Part model, mm, in its own coordinate system. A direction names the side the tool comes from. Coordinates: 2 decimals unless noted, no trailing zeros. Loops run counter-clockwise (first coordinate to the right, second up) from the corner with the lowest first, then second, coordinate; pieces in that order, holes last. Notation, with made-up numbers: (6.5, -14.75) -> (31.5, -14.75) arc R26 cw to (31.5, -0.75) -> close; hole circle Ø7 at (-19, 72). An arc over 180 degrees is marked (long way). One line per question, with ' | ' between items. Start each with the question number.
1) Drop flat-ended pins along their axis: pin 1 (7.5 mm diameter, centred on y = 3, z = -0.5, fed in from -X); pin 2 (5 mm diameter, centred on x = 31, z = 0, fed in from +Y); pin 3 (4 mm diameter, centred on x = 14, z = -33, fed in from -Y); pin 4 (3.5 mm diameter, centred on x = 13.5, y = -12, fed in from -Z). Give the stop position or say it passes through.
2) Cut at C-C (x = -17.5). List the corners of the cut face in (y, z).
3) Cut at A-A (x = 0). List the corners of the cut face in (y, z), plus the area to 3 significant figures.
4) Cut at D-D (y = -1). List the corners of the cut face in (x, z), plus the area to 3 significant figures.
5) 3-axis set-ups, long thin cutter, end or side, ignore diameter. For faces 1 (the face through (23.5, 3, -42)), 2 (the face through (-32, 10, 5)), 3 (the face through (19.8, 11.51, 9.66)), 4 (the face through (-6, 2, -8)): which of +Z, -Z, +X, -X, +Y, -Y reach the whole face in a straight line?
6) Probe L1, parallel to Y at x = 0, z = -56.35; L2, parallel to X at y = 10, z = -55; L3, parallel to Y at x = 0, z = -39. List the from-to ranges inside material, lowest first. Write a range as from..to.
7) Cut at B-B (z = 6). List the corners of the cut face in (x, y).
8) Two-plate mould, pull along Y, no slides. Class faces 5 (the face through (6, 2, -9)), 6 (the face through (20, 11, -9)), 7 (the face through (0, -6, -58)), 8 (the face through (-12.026, -10.648, -57.535)): released by +Y, released by -Y, zero draft, split by the parting line, or undercut.
from build123d import *

# Parameters (mm, degrees)
SKETCH1_W           = 52
SKETCH1_H           = 24
SKETCH1_R           = 8.25
BOSS_EXTRUDE1_DEPTH = 12
SKETCH2_R           = 1
CUT_EXTRUDE1_DEPTH  = 32.048349393
SKETCH3_R           = 1.75
CUT_EXTRUDE2_DEPTH  = 1
FILLET1_R           = 2.5
CUT_EXTRUDE3_DEPTH  = 5
FILLET2_R           = 0.5
SKETCH6_W           = 10
SKETCH6_H           = 10
SKETCH6_R           = 2
BOSS_EXTRUDE2_DEPTH = 5
FILLET3_R           = 4.6
FILLET4_R           = 3
SKETCH9_W           = 47
SKETCH9_H           = 12
BOSS_EXTRUDE3_DEPTH = 48
SKETCH11_W          = 47
SKETCH11_H          = 5
BOSS_EXTRUDE5_DEPTH = 20
CUT_EXTRUDE5_REACH  = 84.946
SKETCH13_R          = 2
CUT_EXTRUDE6_REACH  = 84.946
SKETCH16_R          = 2


with BuildPart() as part:
    # Sketch1 → Boss-Extrude1 (new body)
    with BuildSketch(Plane(origin=(0, 0, 0), x_dir=(1, 0, 0), z_dir=(0, 1, 0))):
        Rectangle(SKETCH1_W, SKETCH1_H)
        with Locations(Location((12.75, 0, 0), (0, 0, 270))):
            Circle(SKETCH1_R, mode=Mode.SUBTRACT)
        with Locations(Location((-12.75, 0, 0), (0, 0, 270))):
            Circle(SKETCH1_R, mode=Mode.SUBTRACT)
    extrude(amount=BOSS_EXTRUDE1_DEPTH)

    # Sketch2 → Cut-Extrude1 (cut, through all)
    with BuildSketch(Plane(origin=(0, 12, 0), x_dir=(1, 0, 0), z_dir=(0, 1, 0))):
        with Locations(Location((-21.35, 8.85, 0), (0, 0, 270))):
            Circle(SKETCH2_R)
        with Locations(Location((21.35, 8.85, 0), (0, 0, 270))):
            Circle(SKETCH2_R)
        with Locations(Location((21.35, -8.85, 0), (0, 0, 270))):
            Circle(SKETCH2_R)
        with Locations(Location((-21.35, -8.85, 0), (0, 0, 270))):
            Circle(SKETCH2_R)
    extrude(amount=-CUT_EXTRUDE1_DEPTH, mode=Mode.SUBTRACT)

    # Sketch3 → Cut-Extrude2 (cut)
    with BuildSketch(Plane(origin=(0, 12, 0), x_dir=(1, 0, 0), z_dir=(0, 1, 0))):
        with Locations(Location((-21.35, 8.85, 0), (0, 0, 270))):
            Circle(SKETCH3_R)
        with Locations(Location((21.35, 8.85, 0), (0, 0, 270))):
            Circle(SKETCH3_R)
        with Locations(Location((21.35, -8.85, 0), (0, 0, 270))):
            Circle(SKETCH3_R)
        with Locations(Location((-21.35, -8.85, 0), (0, 0, 270))):
            Circle(SKETCH3_R)
    extrude(amount=-CUT_EXTRUDE2_DEPTH, mode=Mode.SUBTRACT)

    # Fillet1
    fillet1_edges = [part.edges().sort_by_distance(p)[0] for p in [
        (26, 6, 12),
        (-26, 6, 12),
        (-26, 6, -12),
        (26, 6, -12),
    ]]
    fillet(fillet1_edges, radius=FILLET1_R)

    # Sketch4 → Cut-Extrude3 (cut)
    with BuildSketch(Plane.XZ):
        Polygon((-6, -5), (-6, -12), (6, -12), (6, -5), (0, -5), align=None)
    extrude(amount=-CUT_EXTRUDE3_DEPTH, mode=Mode.SUBTRACT)

    # Fillet2
    fillet2_edges = [part.edges().sort_by_distance(p)[0] for p in [
        (0, 5, -12),
        (6, 2.5, -12),
        (-6, 2.5, -12),
        (-6, 2.5, -5),
        (6, 5, -8.5),
        (6, 2.5, -5),
        (-6, 5, -8.5),
        (0, 5, -5),
    ]]
    fillet(fillet2_edges, radius=FILLET2_R)

    # Sketch6 → Boss-Extrude2 (add)
    # profile 1 of 2: a face of its own
    with BuildSketch(Plane(origin=(0, 12, 0), x_dir=(1, 0, 0), z_dir=(0, 1, 0))):
        with Locations((-31, 0)):
            Rectangle(SKETCH6_W, SKETCH6_H)
        with Locations(Location((-31, 0, 0), (0, 0, 270))):
            Circle(SKETCH6_R, mode=Mode.SUBTRACT)
    # profile 2 of 2: a face of its own
    with BuildSketch(Plane(origin=(0, 12, 0), x_dir=(1, 0, 0), z_dir=(0, 1, 0))):
        with Locations((31, 0)):
            Rectangle(SKETCH6_W, SKETCH6_H)
        with Locations(Location((31, 0, 0), (0, 0, 90))):
            Circle(SKETCH6_R, mode=Mode.SUBTRACT)
    extrude(amount=-BOSS_EXTRUDE2_DEPTH)

    # Fillet3
    # the kernel refuses this fillet: 4.6 mm, written as the material it adds along each edge
    with BuildSketch(Plane(origin=(26, 12, 5), x_dir=(-5.467859312132584e-05, 0, 0.9999999985051258), z_dir=(0, -1, 0)), Plane(origin=(-26, 12, -5), x_dir=(5.467859312132586e-05, 0, -0.9999999985051258), z_dir=(0, -1, 0))) as fillet3_piece_1:
        with BuildLine():
            CenterArc((4.59974851, -4.599547254), FILLET3_R, 90.80387664, 89.192990507)
            Line((-0.000251483, -4.599295733), (-0.460251482, -4.599270581))
            Line((-0.460251482, -4.599270581), (-0.459999999, 2.5152e-05))
            Line((-0.459999999, 2.5152e-05), (2.5152e-05, 0.459999999))
            ThreePointArc((2.5152e-05, 0.459999999), (4.500025145, 0.459753946), (4.528757551, 0.459954725))
            Line((4.528757551, 0.459954725), (4.535211274, 0))
        make_face()
    extrude(amount=5)
    with BuildSketch(Plane(origin=(-26, 12, 5), x_dir=(5.467859312289258e-05, 0, 0.9999999985051258), z_dir=(0, -1, 0)), Plane(origin=(26, 12, -5), x_dir=(-5.467859312132581e-05, 0, -0.9999999985051258), z_dir=(0, -1, 0))) as fillet3_piece_2:
        with BuildLine():
            CenterArc((4.59974851, 4.599547254), FILLET3_R, 180.003132853, 89.192990507)
            Line((-0.000251483, 4.599295733), (-0.460251482, 4.599270581))
            Line((-0.460251482, 4.599270581), (-0.459999999, -2.5152e-05))
            Line((-0.459999999, -2.5152e-05), (2.5152e-05, -0.459999999))
            ThreePointArc((2.5152e-05, -0.459999999), (4.500025145, -0.459753946), (4.528757551, -0.459954725))
            Line((4.528757551, -0.459954725), (4.535211274, 0))
        make_face()
    extrude(amount=5)

    # Fillet4
    fillet4_edges = [part.edges().sort_by_distance(p)[0] for p in [
        (-36, 9.5, 5),
        (-36, 9.5, -5),
        (36, 9.5, -5),
        (36, 9.5, 5),
    ]]
    fillet(fillet4_edges, radius=FILLET4_R)

    # Sketch9 → Boss-Extrude3 (add)
    with BuildSketch(Plane(origin=(0, 0, -12), x_dir=(-1, 0, 0), z_dir=(0, 0, -1))):
        with Locations((0, 6)):
            Rectangle(SKETCH9_W, SKETCH9_H)
    extrude(amount=BOSS_EXTRUDE3_DEPTH)

    # Sketch11 → Boss-Extrude5 (add)
    with BuildSketch(Plane.XZ):
        with Locations((0, -57.5)):
            Rectangle(SKETCH11_W, SKETCH11_H)
    extrude(amount=BOSS_EXTRUDE5_DEPTH)

    # Sketch13 → Cut-Extrude5 (cut, up to next)
    with BuildSketch(Plane(origin=(0, 0, -60), x_dir=(-1, 0, 0), z_dir=(0, 0, -1)), mode=Mode.PRIVATE) as cut_extrude5_sk1:
        with Locations((0, -12)):
            Circle(SKETCH13_R)
    cut_extrude5_tool1 = extrude(cut_extrude5_sk1.sketch, amount=-CUT_EXTRUDE5_REACH, mode=Mode.PRIVATE) & part.part
    # Sketch13 → Cut-Extrude5 (cut, up to next)
    with BuildSketch(Plane(origin=(0, 0, -60), x_dir=(-1, 0, 0), z_dir=(0, 0, -1)), mode=Mode.PRIVATE) as cut_extrude5_sk2:
        with Locations((-13.5, -12)):
            Circle(SKETCH13_R)
    cut_extrude5_tool2 = extrude(cut_extrude5_sk2.sketch, amount=-CUT_EXTRUDE5_REACH, mode=Mode.PRIVATE) & part.part
    # Sketch13 → Cut-Extrude5 (cut, up to next)
    with BuildSketch(Plane(origin=(0, 0, -60), x_dir=(-1, 0, 0), z_dir=(0, 0, -1)), mode=Mode.PRIVATE) as cut_extrude5_sk3:
        with Locations((13.5, -12)):
            Circle(SKETCH13_R)
    cut_extrude5_tool3 = extrude(cut_extrude5_sk3.sketch, amount=-CUT_EXTRUDE5_REACH, mode=Mode.PRIVATE) & part.part
    add(cut_extrude5_tool1.solids().sort_by_distance((0, -12, -60))[0], mode=Mode.SUBTRACT)
    add(cut_extrude5_tool2.solids().sort_by_distance((13.5, -12, -60))[0], mode=Mode.SUBTRACT)
    add(cut_extrude5_tool3.solids().sort_by_distance((-13.5, -12, -60))[0], mode=Mode.SUBTRACT)

    # Sketch16 → Cut-Extrude6 (cut, up to next)
    with BuildSketch(Plane(origin=(0, 0, -60), x_dir=(-1, 0, 0), z_dir=(0, 0, -1)), mode=Mode.PRIVATE) as cut_extrude6_sk1:
        with Locations((0, -4)):
            Circle(SKETCH16_R)
    cut_extrude6_tool1 = extrude(cut_extrude6_sk1.sketch, amount=-CUT_EXTRUDE6_REACH, mode=Mode.PRIVATE) & part.part
    add(cut_extrude6_tool1.solids().sort_by_distance((0, -4, -60))[0], mode=Mode.SUBTRACT)


solid = part.part
Reported:
1) pin 1: stops at x = -26 | pin 2: stops at y = 12 | pin 3: stops at y = 0 | pin 4: passes through
2) outline: (-20, -60) -> (12, -60) -> (12, -6.75) -> (0, -6.75) -> (0, -55) -> (-20, -55) -> close; (0, 6.75) -> (12, 6.75) -> (12, 12) -> (0, 12) -> close
3) outline: (-20, -60) -> (-14, -60) -> (-14, -55) -> (-20, -55) -> close; (-10, -60) -> (-6, -60) -> (-6, -55) -> (-10, -55) -> close; (-2, -60) -> (12, -60) -> (12, 12) -> (0, 12) -> (0, -5) -> (4.5, -5) arc R0.5 cw to (5, -5.5) -> (5, -11.5) arc R0.5 ccw to (5.5, -12) -> (0, -12) -> (0, -55) -> (-2, -55) -> close | area: 889 mm²
4) outline: (-23.5, -60) -> (23.5, -60) -> (23.5, -55) -> (-23.5, -55) -> close | area: 235 mm²
5) face 1: -Z, +X, +Y, -Y | face 2: +Z, -X, +Y, -Y | face 3: +Y | face 4: -Y
6) L1: y = -20..-14, -10..-6, -2..12 | L2: x = -23.5..23.5 | L3: y = 0..12
7) outline: (-27.74, 7) -> (-26, 7) -> (-26, 0) -> (-18.41, 0) -> (-18.41, 12) -> (-27.74, 12) -> close; (-7.09, 0) -> (7.09, 0) -> (7.09, 12) -> (-7.09, 12) -> close; (18.41, 0) -> (26, 0) -> (26, 7) -> (27.74, 7) -> (27.74, 12) -> (18.41, 12) -> close
8) face 5: zero draft | face 6: released by +Y | face 7: undercut | face 8: undercut
